Check sheet for the modelled part. Datum: model origin and axes. Units: mm. Give positions to 0.01 mm unless a question says otherwise; leave off trailing zeros. Order: outer loops, then holes, each group sorted by start corner. A loop starts at its lowest first (then second) coordinate and runs counter-clockwise, first axis right, second up.
```python
from build123d import *

# Parameters (mm, degrees)
SKETCH1_W                                  = 175
SKETCH1_H                                  = 50
BOSS_EXTRUDE1_DEPTH                        = 2
BOSS_EXTRUDE2_START                        = 11
SKETCH2_W                                  = 175
SKETCH2_H                                  = 50
BOSS_EXTRUDE2_DEPTH                        = 2
BOSS_EXTRUDE3_START                        = 5
SKETCH3_W                                  = 175
SKETCH3_H                                  = 50
BOSS_EXTRUDE3_DEPTH                        = 2
SKETCH5_W                                  = 160
SKETCH5_H                                  = 40
BOSS_EXTRUDE4_DEPTH                        = 10
SKETCH7_W                                  = 5
SKETCH7_H                                  = 35
CUT_EXTRUDE1_DEPTH                         = 0.1
LPATTERN1_COUNT                            = 16
LPATTERN1_PITCH                            = 10
SKETCH8_R                                  = 2.5
BOSS_EXTRUDE5_DEPTH                        = 18
MIRROR1_AT_THE_SECOND_PLANE_COPY_1_SKETC_R = 2.5
MIRROR1_AT_THE_SECOND_PLANE_COPY_1_DEPTH   = 18
FILLET2_R                                  = 2.75


with BuildPart() as part:
    # Sketch1 → Boss-Extrude1 (new body)
    with BuildSketch(Plane(origin=(0, 0, 0), x_dir=(1, 0, 0), z_dir=(0, 1, 0))):
        Rectangle(SKETCH1_W, SKETCH1_H)
    extrude(amount=BOSS_EXTRUDE1_DEPTH)

    # Sketch5 → Boss-Extrude4 (add)
    with BuildSketch(Plane(origin=(0, 2, 0), x_dir=(1, 0, 0), z_dir=(0, 1, 0))):
        Rectangle(SKETCH5_W, SKETCH5_H)
    extrude(amount=BOSS_EXTRUDE4_DEPTH)

    # Sketch7 → Cut-Extrude1 (cut)
    with BuildSketch(Plane(origin=(0, 12, 0), x_dir=(1, 0, 0), z_dir=(0, 1, 0))):
        with Locations((-75, 0)):
            Rectangle(SKETCH7_W, SKETCH7_H)
    cut_extrude1 = extrude(amount=-CUT_EXTRUDE1_DEPTH, mode=Mode.SUBTRACT)

    # LPattern1: Cut-Extrude1 ×16
    with Locations(*[(i * LPATTERN1_PITCH, 0, 0) for i in range(1, LPATTERN1_COUNT)]):
        add(cut_extrude1, mode=Mode.SUBTRACT)



with BuildPart() as body_2:
    # Sketch2 → Boss-Extrude2 (new body)
    with BuildSketch(Plane(origin=(0, 2, 0), x_dir=(1, 0, 0), z_dir=(0, 1, 0)).offset(BOSS_EXTRUDE2_START)):
        Rectangle(SKETCH2_W, SKETCH2_H)
    extrude(amount=BOSS_EXTRUDE2_DEPTH)


with BuildPart() as body_3:
    # Sketch3 → Boss-Extrude3 (new body)
    with BuildSketch(Plane.XZ.offset(BOSS_EXTRUDE3_START)):
        Rectangle(SKETCH3_W, SKETCH3_H)
    extrude(amount=BOSS_EXTRUDE3_DEPTH)


with BuildPart() as part_1:
    add(part.part)

    add(body_2.part)  # Boss-Extrude5 merges body 2

    add(body_3.part)  # Boss-Extrude5 merges body 3
    # Sketch8 → Boss-Extrude5 (add)
    with BuildSketch(Plane(origin=(0, -5, 0), x_dir=(1, 0, 0), z_dir=(0, 1, 0))):
        with Locations((-84.75, 22.25)):
            Circle(SKETCH8_R)
    boss_extrude5 = extrude(amount=BOSS_EXTRUDE5_DEPTH)

    # Mirror1: Boss-Extrude5 across plane
    add(boss_extrude5.mirror(Plane(origin=(0, 0, 0), x_dir=(0, 0, 1), z_dir=(1, 0, 0))))

    # Mirror1 at the second plane: Boss-Extrude5 across plane
    add(boss_extrude5.mirror(Plane.XY))

    # Mirror1 at the second plane copy 1 sketc → Mirror1 at the second plane copy 1 (add)
    with BuildSketch(Plane(origin=(0, -5, 0), x_dir=(-1, 0, 0), z_dir=(0, 1, 0))):
        with Locations((-84.75, 22.25)):
            Circle(MIRROR1_AT_THE_SECOND_PLANE_COPY_1_SKETC_R)
    extrude(amount=MIRROR1_AT_THE_SECOND_PLANE_COPY_1_DEPTH)

    # Fillet2
    fillet2_edges = [part_1.edges().sort_by_distance(p)[0] for p in [
        (87.5, -6, 25),
        (-87.5, -6, 25),
        (-87.5, -6, -25),
        (87.5, -6, -25),
        (-87.5, 1, -25),
        (-87.5, 1, 25),
        (87.5, 1, 25),
        (87.5, 1, -25),
        (87.5, 14, -25),
        (87.5, 14, 25),
        (-87.5, 14, 25),
        (-87.5, 14, -25),
    ]]
    fillet(fillet2_edges, radius=FILLET2_R)


solid = part_1.part
```
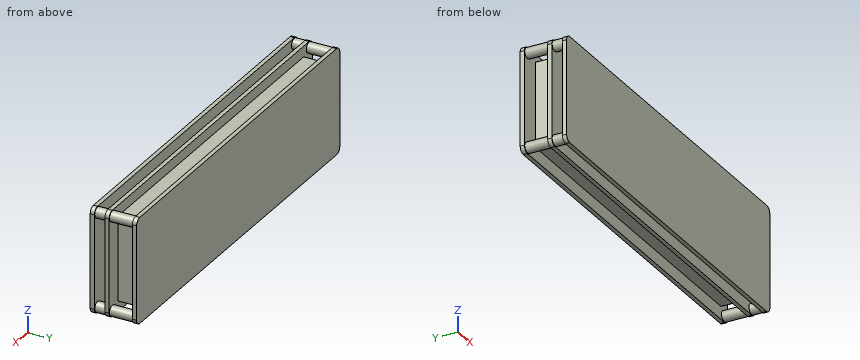
(1) Sectioned sample at B-B (z = 5.5). Count the separate pieces of the cut face and the enclosed holes in it, plus the area to 3 significant figures.
(2) Sectioned sample at A-A (y = 9). Enter the section's corners in (x, z), plus the area to 3 significant figures.
(3) Thickness scan on L1, parallel to Y at x = 62, z = -10.5; L2, parallel to Y at x = -3, z = -4.5; L3, parallel to X at y = 7, z = -15.5. Record the ranges inside material, lowest first.
(4) Go/stop test with flat-tipped pins: P1, Ø5, axis at x = 12.5, y = 2.5, coming from the +Z side; P2, Ø1.5, axis at x = 10.5, y = 11.5, coming from the -Z side; P3, Ø2, axis at x = -10.5, y = 7, coming from the +Z side. Record where each tip stops, or that it passes through.
Values follow:
1. separate pieces: 3
1. enclosed holes: 0
1. area: 2,640 mm2
2. outline: circle Ø5 at (-84.75, -22.25); circle Ø5 at (-84.75, 22.25); (-80, -20) - (80, -20) - (80, 20) - (-80, 20) - close; circle Ø5 at (84.75, -22.25); circle Ø5 at (84.75, 22.25)
2. area: 6,480 mm2
3. L1: y = -7 to -5, 0 to 12, 13 to 15
3. L2: y = -7 to -5, 0 to 11.9, 13 to 15
3. L3: x = -80 to 80
4. P1: stops at z = 25
4. P2: stops at z = -20
4. P3: stops at z = 20
